from build123d import *

# Parameters (mm, degrees)
F0_W     = 15
F0_H     = 28
F1_DEPTH = 2
F2_R     = 7
F3_R     = 1
F4_DEPTH = 2


with BuildPart() as f1:
    # F0 (on Top) → F1 (new body)
    with BuildSketch(Plane.XY):
        Rectangle(F0_W, F0_H)
    extrude(amount=F1_DEPTH)

    # F2
    f2_edges = [f1.edges().sort_by_distance(p)[0] for p in [
        (-7.5, -14, 1),
        (7.5, -14, 1),
    ]]
    fillet(f2_edges, radius=F2_R)

    # F3 (on face) → F4 (cut, through all)
    with BuildSketch(Plane.XY.offset(2)):
        with BuildLine():
            ThreePointArc((0, -10.5), (1.767767, -9.767767), (2.5, -8))
            ThreePointArc((2.5, -8), (-1.767767, -6.232233), (0, -10.5))
        make_face()
        with Locations((0, 5)):
            Circle(F3_R)
        with Locations((0, 11)):
            Circle(F3_R)
    extrude(amount=-F4_DEPTH, mode=Mode.SUBTRACT)


solid = f1.part
The listing builds one solid part. Answer for the finished solid, in the listing's coordinates (mm). Coordinates: 2 decimals unless noted, no trailing zeros. Order: outer loops, then holes, each group sorted by start corner. A loop starts at its lowest first (then second) coordinate and runs counter-clockwise, first axis right, second up.
Q1. A cutting plane is placed at B-B, the plane y = 11. Write down the section's boundary in (x, z), and give its area (3 significant figures).
Q2. Given P1, Ø3, axis at x = 0, y = 11, coming from the -Z side; P2, Ø1.6, axis at x = 0, y = 5, coming from the -Z side, each flat-ended and moving along its own axis, determine where each tip first touches the part or whether it passes through.
Q3. A cutting plane is placed at D-D, the plane x = 6.5. Write down the section's boundary in (y, z), and give its area (3 significant figures).
Q4. For a pull along X with two mould halves and no side action, classify faces 1 (the face through (-7.5, 3, 1)), 2 (the face through (5.4, -12, 1)), 3 (the face through (0, 6, 1)) as pulls with the +X half, pulls with the -X half, needs draft (parallel to the pull), parting line crosses it, or undercut.
Q5. Consider line 1 (Y direction, x = 0, z = 1.45); line 2 (Y direction, x = -0.5, z = 0.9); line 3 (Y direction, x = -1.5, z = 0.2). Determine where each line is inside the solid, lowest interval first.
Q6. A cutting plane is placed at A-A, the plane z = 1.7. Write down the section's boundary in (x, y).
Q7. A cutting plane is placed at C-C, the plane y = -10. Write down the section's boundary in (x, z).
Answers follow:
1. outline: (-7.5, 0) - (-1, 0) - (-1, 2) - (-7.5, 2) - close; (1, 0) - (7.5, 0) - (7.5, 2) - (1, 2) - close
1. area: 26.0 mm2
2. P1: stops at z = 0
2. P2: passes through
3. outline: (-10.61, 0) - (14, 0) - (14, 2) - (-10.61, 2) - close
3. area: 49.2 mm2
4. face 1: pulls with the -X half
4. face 2: pulls with the +X half
4. face 3: undercut
5. line 1: y = -14 to -10.5, -5.5 to 4, 6 to 10, 12 to 14
5. line 2: y = -14 to -10.45, -5.55 to 4.13, 5.87 to 10.13, 11.87 to 14
5. line 3: y = -13.93 to -10, -6 to 14
6. outline: (-7.5, -7) arc R7 ccw to (-0.5, -14) - (0.5, -14) arc R7 ccw to (7.5, -7) - (7.5, 14) - (-7.5, 14) - close; hole circle Ø5 at (0, -8); hole circle Ø2 at (0, 5); hole circle Ø2 at (0, 11)
7. outline: (-6.82, 0) - (-1.5, 0) - (-1.5, 2) - (-6.82, 2) - close; (1.5, 0) - (6.82, 0) - (6.82, 2) - (1.5, 2) - close
